```python
from build123d import *

# Parameters (mm, degrees)
STOCK_BACK_1_OUTLINE_W = 12.9
STOCK_BACK_1_OUTLINE_H = 19
STOCK_BACK_1_DEPTH     = 6
SKETCH2_W              = 28.3
SKETCH2_H              = 3
BOSS_EXTRUDE2_DEPTH    = 6
LPATTERN2_COUNT        = 5
LPATTERN2_PITCH        = 111
SKETCH3_W              = 116
SKETCH3_H              = 6
BOSS_EXTRUDE4_DEPTH    = 6
CUT_EXTRUDE1_DEPTH     = 3


# Read off the part's stored shape, not the designer's step: Stock-Back-1
with BuildPart() as part:
    # Stock-Back-1 outline → Stock-Back-1 (new body)
    with BuildSketch(Plane.XY):
        with BuildLine():
            Line((0, 457), (0, 366))
            Line((0, 366), (500, 366))
            Line((500, 366), (500, 457))
            ThreePointArc((500, 457), (487.112698372, 488.112698372), (456, 501))
            Line((456, 501), (44, 501))
            ThreePointArc((44, 501), (12.887301628, 488.112698372), (0, 457))
        make_face()
        with Locations((449.55, 421)):
            Rectangle(STOCK_BACK_1_OUTLINE_W, STOCK_BACK_1_OUTLINE_H, mode=Mode.SUBTRACT)
    extrude(amount=STOCK_BACK_1_DEPTH)

    # Sketch2 → Boss-Extrude2 (add)
    with BuildSketch(Plane(origin=(0, 0, 0), x_dir=(-1, 0, 0), z_dir=(0, 0, -1))):
        with Locations((-472.2, 364.5)):
            Rectangle(SKETCH2_W, SKETCH2_H)
    boss_extrude2 = extrude(amount=-BOSS_EXTRUDE2_DEPTH)

    # LPattern2: Boss-Extrude2 ×5
    with Locations(*[(-i * LPATTERN2_PITCH, 0, 0) for i in range(1, LPATTERN2_COUNT)]):
        add(boss_extrude2)

    # Sketch3 → Boss-Extrude4 (add)
    with BuildSketch(Plane(origin=(0, 0, 0), x_dir=(-1, 0, 0), z_dir=(0, 0, -1))):
        with Locations((-250, 504)):
            Rectangle(SKETCH3_W, SKETCH3_H)
    extrude(amount=-BOSS_EXTRUDE4_DEPTH)

    # Sketch4 → Cut-Extrude1 (cut)
    with BuildSketch(Plane(origin=(0, 507, 0), x_dir=(1, 0, 0), z_dir=(0, 1, 0))):
        with BuildLine():
            Line((219, -6), (281, -6))
            Line((281, -6), (281, -5))
            ThreePointArc((281, -5), (280.414213562, -3.585786438), (279, -3))
            Line((279, -3), (221, -3))
            ThreePointArc((221, -3), (219.585786438, -3.585786438), (219, -5))
            Line((219, -5), (219, -6))
        make_face()
        with BuildLine():
            Line((219, -3), (219, -5))
            ThreePointArc((219, -5), (219.585786438, -3.585786438), (221, -3))
            Line((221, -3), (219, -3))
        make_face()
        with BuildLine():
            ThreePointArc((279, -3), (280.414213562, -3.585786438), (281, -5))
            Line((281, -5), (281, -3))
            Line((281, -3), (279, -3))
        make_face()
    extrude(amount=-CUT_EXTRUDE1_DEPTH, mode=Mode.SUBTRACT)


solid = part.part
```
Could you check a few things on this model? Use its own coordinates, in mm. Give positions to 0.01 mm unless a question says otherwise; leave off trailing zeros. Order: outer loops, then holes, each group sorted by start corner. A loop starts at its lowest first (then second) coordinate and runs counter-clockwise, first axis right, second up.
Q1. If I drill on line 1 along X through (y, z) = (414, 5.5); line 2 along X through (y, z) = (458, 1.8); line 3 along Y through (x, z) = (75.5, 0.9), over which ranges is the centre line in solid material (lowest first)?
Q2. Suppose I cut it at C-C, the plane x = 272. Write out the boundary of the cut face in (y, z).
Q3. Suppose I cut it at D-D, the plane y = 481. Write out the boundary of the cut face in (x, z), and give its area (3 significant figures).
Q4. I'm going to push flat-ended pins straight in: P1, Ø2.5, axis at y = 506, z = 4.5, coming from the +X side; P2, Ø3, axis at y = 505.5, z = 1.5, coming from the -X side; P3, Ø1.5, axis at x = 242, z = 4, coming from the +Y side. Where does each tip first touch, or does it pass through?
Q5. Suppose I cut it at A-A, the plane y = 421.5. Write out the boundary of the cut face in (x, z), and give its area (3 significant figures).
Solution:
1. line 1: x = 0 to 443.1, 456 to 500
1. line 2: x = 0.01 to 499.99
1. line 3: y = 366 to 501
2. outline: (366, 0) - (507, 0) - (507, 3) - (504, 3) - (504, 6) - (366, 6) - close
3. outline: (7.12, 0) - (492.88, 0) - (492.88, 6) - (7.12, 6) - close
3. area: 2,910 mm2
4. P1: stops at x = 308
4. P2: stops at x = 192
4. P3: stops at y = 504
5. outline: (0, 0) - (443.1, 0) - (443.1, 6) - (0, 6) - close; (456, 0) - (500, 0) - (500, 6) - (456, 6) - close
5. area: 2,920 mm2
